Build history of the part. All positions in model axes, mm. Face numbers are marked on the shaded views. A direction names the side the tool comes from. Round coordinates to 2 decimals unless told otherwise and drop trailing zeros. Loops run counter-clockwise (first coordinate to the right, second up) from the corner with the lowest first, then second, coordinate; pieces in that order, holes last.
from build123d import *

# Parameters (mm, degrees)
SKETCH1_W           = 5.5
SKETCH1_H           = 5
BOSS_EXTRUDE1_DEPTH = 7.5
CUT_EXTRUDE1_DEPTH  = 2
CUT_EXTRUDE2_DEPTH  = 1
CUT_EXTRUDE3_DEPTH  = 2
CUT_EXTRUDE4_DEPTH  = 2
SKETCH6_W           = 2.5
SKETCH6_H           = 4
CUT_EXTRUDE5_DEPTH  = 1
SKETCH7_W           = 1
SKETCH7_H           = 2
CUT_EXTRUDE6_DEPTH  = 5
SKETCH8_W           = 2
SKETCH8_H           = 1
CUT_EXTRUDE7_DEPTH  = 6.5
CUT_EXTRUDE8_DEPTH  = 4
SKETCH11_W          = 1.5
SKETCH11_H          = 1.5
CUT_EXTRUDE9_DEPTH  = 1.5


with BuildPart() as part:
    # Sketch1 → Boss-Extrude1 (new body)
    with BuildSketch(Plane.XY):
        Rectangle(SKETCH1_W, SKETCH1_H)
    extrude(amount=BOSS_EXTRUDE1_DEPTH)

    # Sketch2 → Cut-Extrude1 (cut)
    with BuildSketch(Plane.ZY.offset(2.75)):
        Polygon((6, 2.5), (7.5, -1.5), (7.5, 2.5), align=None)
    extrude(amount=-CUT_EXTRUDE1_DEPTH, mode=Mode.SUBTRACT)

    # Sketch3 → Cut-Extrude2 (cut)
    with BuildSketch(Plane(origin=(2.75, 0, 0), x_dir=(0, 0, -1), z_dir=(1, 0, 0))):
        Polygon((0, -2.5), (-2, -2.5), (-2, 0.5), (-4, 0.5), (-4, 2.5), (0, 2.5), align=None)
    extrude(amount=-CUT_EXTRUDE2_DEPTH, mode=Mode.SUBTRACT)

    # Sketch4 → Cut-Extrude3 (cut)
    with BuildSketch(Plane(origin=(0, 2.5, 0), x_dir=(1, 0, 0), z_dir=(0, 1, 0))):
        Polygon((2.75, -7.5), (2.75, -4), (1.75, -4), (-2.75, -4), (-2.75, -6), (-0.75, -6), (-0.75, -7.5), align=None)
    extrude(amount=-CUT_EXTRUDE3_DEPTH, mode=Mode.SUBTRACT)

    # Sketch5 → Cut-Extrude4 (cut)
    with BuildSketch(Plane.ZY.offset(2.75)):
        Polygon((6, 2.5), (6, 0.5), (7.5, -1.5), align=None)
    extrude(amount=-CUT_EXTRUDE4_DEPTH, mode=Mode.SUBTRACT)

    # Sketch6 → Cut-Extrude5 (cut)
    with BuildSketch(Plane(origin=(0, 2.5, 0), x_dir=(1, 0, 0), z_dir=(0, 1, 0))):
        Polygon((1.75, -4), (1.75, -1), (0.75, -4), align=None)
        with Locations((-1.5, -2)):
            Rectangle(SKETCH6_W, SKETCH6_H)
    extrude(amount=-CUT_EXTRUDE5_DEPTH, mode=Mode.SUBTRACT)

    # Sketch7 → Cut-Extrude6 (cut, through all)
    with BuildSketch(Plane(origin=(0, 1.5, 0), x_dir=(1, 0, 0), z_dir=(0, 1, 0))):
        with Locations((-2.25, -1)):
            Rectangle(SKETCH7_W, SKETCH7_H)
    extrude(amount=-CUT_EXTRUDE6_DEPTH, mode=Mode.SUBTRACT)

    # Sketch8 → Cut-Extrude7 (cut, through all)
    with BuildSketch(Plane(origin=(2.75, 0, 0), x_dir=(0, 0, -1), z_dir=(1, 0, 0))):
        with Locations((-4, -2)):
            Rectangle(SKETCH8_W, SKETCH8_H)
    extrude(amount=-CUT_EXTRUDE7_DEPTH, mode=Mode.SUBTRACT)

    # Sketch10 → Cut-Extrude8 (cut, through all)
    with BuildSketch(Plane(origin=(0, 0.5, 0), x_dir=(1, 0, 0), z_dir=(0, 1, 0))):
        Polygon((2.75, -6), (1.25, -7.5), (2.75, -7.5), align=None)
    extrude(amount=-CUT_EXTRUDE8_DEPTH, mode=Mode.SUBTRACT)

    # Sketch11 → Cut-Extrude9 (cut)
    with BuildSketch(Plane(origin=(2.75, 0, 0), x_dir=(0, 0, -1), z_dir=(1, 0, 0))):
        with Locations((-6.75, -1.75)):
            Rectangle(SKETCH11_W, SKETCH11_H)
    extrude(amount=-CUT_EXTRUDE9_DEPTH, mode=Mode.SUBTRACT)


solid = part.part
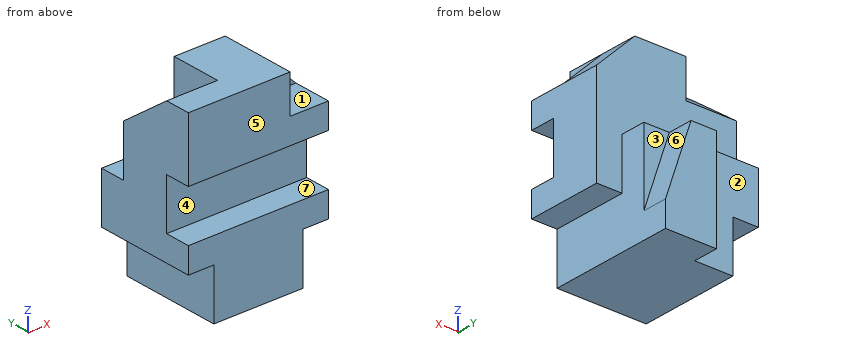
(1) Probe line 1 (Z direction, x = 1.15, y = -2); line 2 (Z direction, x = 0.85, y = 1.4); line 3 (Y direction, x = 0.75, z = 3.25). List the from-to ranges inside material, lowest first.
Responses:
line 1: z = 0 to 3, 5 to 7.5
line 2: z = 0 to 4
line 3: y = -1.5 to 2.5
(2) Which spindle directions (+Z, -Z, +X, -X, +Y, -Y) get a long thin tool onto all of the face, cutting with end or side? Do the marked faces 1, 2, 3 and 4. Say none if no direction does.
Responses:
face 1: +Z, +X, -Y
face 2: +Z, -Z, -X, +Y
face 3: +Z, +X, +Y
face 4: +X, -X, -Y
(3) Slice it at B-B on z = 2.5. List the corners of the cut face in (x, y), plus the area to 3 significant figures.
Responses:
outline: (-2.75, -2.5) - (2.75, -2.5) - (2.75, 0.5) - (1.75, 0.5) - (1.75, 1.5) - (1.25, 1.5) - (1.25, 2.5) - (-0.25, 2.5) - (-0.25, 1.5) - (-2.75, 1.5) - close
area: 22.5 mm2
(4) Pin check, flat tips, straight feed: P1, Ø1.5, axis at x = -0.5, z = 5, coming from the +Y side; P2, Ø1.2, axis at x = 2, z = 7, coming from the -Y side; P3, Ø0.6, axis at y = -0.5, z = 1, coming from the -X side. Stop position of each tip, or through.
Responses:
P1: stops at y = 0.5
P2: stops at y = -1
P3: stops at x = -1.75
(5) Slice it at D-D on y = 1.7. List the corners of the cut face in (x, z).
Responses:
outline: (-0.25, 0) - (1.75, 0) - (1.75, 1) - (0.75, 4) - (-0.25, 4) - close
(6) Pull direction Z, two halves, no side cores. Call the marked faces 5, 6 and 7: +Z half, -Z half, draft (parallel to the pull), parting line (faces both ways), or undercut.
Responses:
face 5: draft
face 6: +Z half
face 7: undercut
(7) Slice it at A-A on y = -2.1. List the corners of the cut face in (x, z).
Responses:
outline: (-2.75, 2) - (-1.75, 2) - (-1.75, 0) - (1.75, 0) - (1.75, 2) - (2.75, 2) - (2.75, 3) - (-2.75, 3) - close; (-2.75, 5) - (2.75, 5) - (2.75, 6) - (1.25, 6) - (1.25, 7.5) - (-2.75, 7.5) - close
(8) Slice it at C-C on x = 1.45. List the corners of the cut face in (y, z), plus the area to 4 significant figures.
Responses:
outline: (-2.5, 0) - (2.5, 0) - (2.5, 1.9) - (1.5, 1.9) - (1.5, 4) - (0.5, 4) - (0.5, 7.3) - (-1, 7.3) - (-1, 6) - (-2.5, 6) - (-2.5, 5) - (-1.5, 5) - (-1.5, 3) - (-2.5, 3) - close
area: 23.85 mm2
